Verification items for the finished model (mm, model axes). A direction names the side the tool comes from. Coordinates: 2 decimals unless noted, no trailing zeros. Order: outer loops, then holes, each group sorted by start corner. A loop starts at its lowest first (then second) coordinate and runs counter-clockwise, first axis right, second up. Notation, with made-up numbers: M 39,75 L 45,75 A5 cw 45,83 Z; hole C 33.25,-14 d4. An arc over 180 degrees is marked long. Return JSON: item names as keys, results as strings. Group by question number.
1. Gauge pin test, flat ends, axial feed: pin 1 (17.5 mm diameter, centred on x = 743.5, z = 33.5, fed in from +Y); pin 2 (3 mm diameter, centred on x = 438.5, z = 57, fed in from -Y); pin 3 (1.5 mm diameter, centred on x = 459, y = 62.5, fed in from +Z); pin 4 (3 mm diameter, centred on x = 397, y = 9, fed in from +Z). Record the tip position at first contact, or that the pin passes through.
2. Set-up check for faces 4 (the cylindrical face through (1201.241, 5.916, 34.924)), 5 (the flat face through (701, 41, 12)): record each of +Z, -Z, +X, -X, +Y, -Y from which the full face is reachable in a straight line by a thin tool's end or side.
3. Mould release check, pull along X, two halves, no side actions. Record for faces 1 (the flat face through (0, 25, 10)), 2 (the flat face through (701, 12, 47)), 3 (the cylindrical face through (1376.508, 43.304, 5.916)): +X half, -X half, draft (parallel to the pull), parting line (faces both ways), or undercut.
4. Material ranges on line 1 along Y through (x, z) = (1299.5, 56); line 2 along Z through (x, y) = (711, 8.25), recorded low to high.
5. Section check A-A, the plane x = 864.5. Record the cut outline in (y, z), plus the area to 3 significant figures.
```python
from build123d import *

# Parameters (mm, degrees)
SKETCH_1_W             = 1422
SKETCH_1_H             = 80
EXTRUDE_1_DEPTH        = 80
SKETCH_3_W             = 68
SKETCH_3_H             = 68
CUT_EXTRUDE_2_DEPTH    = 1427.49360321
FILLET_1_R             = 10
SKETCH_4_R             = 11
CUT_EXTRUDE_3_DEPTH    = 1427.49360321
PATTERN_LINEAR_1_COUNT = 2
PATTERN_LINEAR_1_PITCH = 1352
SKETCH_5_R             = 11
CUT_EXTRUDE_4_DEPTH    = 1427.49360321
PATTERN_LINEAR_2_COUNT = 11
PATTERN_LINEAR_2_PITCH = 125


with BuildPart() as part:
    # 草图1 → 拉伸1 (new body)
    with BuildSketch(Plane.XY):
        with Locations((711, 40)):
            Rectangle(SKETCH_1_W, SKETCH_1_H)
    extrude(amount=EXTRUDE_1_DEPTH)

    # 草图3 → 拉伸2 (cut, through all)
    with BuildSketch(Plane.ZY):
        with Locations((46, 46)):
            Rectangle(SKETCH_3_W, SKETCH_3_H)
    extrude(amount=-CUT_EXTRUDE_2_DEPTH, mode=Mode.SUBTRACT)

    # 圆角1
    fillet_1_edges = [part.edges().sort_by_distance(p)[0] for p in [
        (711, 80, 12),
        (711, 12, 80),
    ]]
    fillet(fillet_1_edges, radius=FILLET_1_R)

    # 草图4 → 拉伸3 (cut, through all)
    with BuildSketch(Plane(origin=(0, 0, 0), x_dir=(-1, 0, 0), z_dir=(0, 0, -1))):
        with Locations((-1387, 40)):
            Circle(SKETCH_4_R)
    cut_extrude_3 = extrude(amount=-CUT_EXTRUDE_3_DEPTH, mode=Mode.SUBTRACT)

    # 阵列(线性)1: 拉伸3 ×2
    with Locations(*[(-i * PATTERN_LINEAR_1_PITCH, 0, 0) for i in range(1, PATTERN_LINEAR_1_COUNT)]):
        add(cut_extrude_3, mode=Mode.SUBTRACT)

    # 草图5 → 拉伸4 (cut, through all)
    with BuildSketch(Plane.XZ):
        with Locations(Location((86, 40, 0), (0, 0, 270))):
            Circle(SKETCH_5_R)
    cut_extrude_4 = extrude(amount=-CUT_EXTRUDE_4_DEPTH, mode=Mode.SUBTRACT)

    # 阵列(线性)2: 拉伸4 ×11
    with Locations(*[(i * PATTERN_LINEAR_2_PITCH, 0, 0) for i in range(1, PATTERN_LINEAR_2_COUNT)]):
        add(cut_extrude_4, mode=Mode.SUBTRACT)


solid = part.part
```
Answers follow:
{
 "1": {"pin 1": "y = 12", "pin 2": "y = 0", "pin 3": "z = 12", "pin 4": "z = 78.35"},
 "2": {"face 4": "+Y, -Y", "face 5": "+Z, +X, -X, +Y"},
 "3": {"face 1": "-X half", "face 2": "draft", "face 3": "undercut"},
 "4": {"line 1": "0 to 12", "line 2": "0 to 29, 51 to 77.81"},
 "5": {"outline": "M 0,0 L 80,0 L 80,2 A10 ccw 70,12 L 12,12 L 12,70 A10 ccw 2,80 L 0,80 Z", "area": "1,730 mm^2"}
}
